Read the model definition and answer for the solid it produces. Units are mm, in the model's axes. Coordinates: 2 decimals unless noted, no trailing zeros. Order: outer loops, then holes, each group sorted by start corner. A loop starts at its lowest first (then second) coordinate and runs counter-clockwise, first axis right, second up. Notation, with made-up numbers: (64.25, 87) -> (112.25, 87) arc R31 ccw to (112.25, 115) -> close; hole circle Ø1 at (70.25, -30.75). An arc over 180 degrees is marked (long way). Answer in a Markdown table with one row per item.
from build123d import *

# Parameters (mm, degrees)
REVOLVE3_ANGLE      = 90
BOSS_EXTRUDE2_DEPTH = 1000


with BuildPart() as part:
    # Sketch2 → Revolve3 (revolve)
    with BuildSketch(Plane.XY):
        with BuildLine():
            Line((-0.654182434, 15.02), (-10.654182434, 15.02))
            Line((-10.654182434, 15.02), (-10.654182434, 0))
            Line((-10.654182434, 0), (0, 0))
            Line((0, 0), (25.4, 0))
            Line((25.4, 0), (35.4, 0))
            Line((35.4, 0), (35.4, 4.5))
            Line((35.4, 4.5), (25.4, 4.5))
            add(Edge.make_bspline(
                [(-0.654182434, 15.02), (-0.219836229, 14.810704372), (0.610598489, 14.410982375), (2.74095302, 13.386545583), (4.34709547, 12.619135975), (6.701613478, 11.49599419), (8.606916476, 10.59589253), (10.790885987, 9.570629713), (12.810835282, 8.63757915), (14.944119423, 7.669787097), (16.950761864, 6.79193378), (18.75556814, 6.044207346), (20.238794329, 5.486207444), (21.39416777, 5.103578745), (22.215591012, 4.870934478), (22.897035956, 4.710298297), (23.464492683, 4.605633048), (23.954091395, 4.538072471), (24.354277235, 4.503624983), (24.669284768, 4.488813447), (24.918595629, 4.485402054), (25.124701431, 4.488218611), (25.279381224, 4.493757229), (25.359889237, 4.497669109), (25.4, 4.5)],
                knots=[0.083771138, 0.083771138, 0.083771138, 0.083771138, 0.083771138, 0.152014176, 0.220257214, 0.288500251, 0.356743288, 0.424986327, 0.493229366, 0.561472406, 0.629715448, 0.697958493, 0.757156968, 0.791278497, 0.81934393, 0.841893906, 0.858954658, 0.874282948, 0.887931591, 0.900718778, 0.906405686, 0.912092593, 0.917779499, 0.923466404, 0.923466404, 0.923466404, 0.923466404, 0.923466404], degree=4))
        make_face()
    revolve(axis=Axis((0, 0, 0), (1, 0, 0)), revolution_arc=REVOLVE3_ANGLE)

    # Sketch11 → Boss-Extrude2 (add)
    with BuildSketch(Plane.XY):
        with BuildLine():
            Line((25.133318649, 0), (101.333318649, 0))
            ThreePointArc((101.333318649, 0), (63.233318649, 38.1), (25.133318649, 0))
        make_face()
    extrude(amount=BOSS_EXTRUDE2_DEPTH)


solid = part.part
Q1. Given pin 1 (5 mm diameter, centred on y = 6, z = 335.5, fed in from +X); pin 2 (12 mm diameter, centred on x = 67.5, z = 570.5, fed in from +Y); pin 3 (8 mm diameter, centred on x = 52, z = 739.5, fed in from +Y), each flat-ended and moving along its own axis, determine where each tip first touches the part or whether it passes through.
Outcome:
| item | result |
|---|---|
| pin 1 | x = 101.17 |
| pin 2 | y = 38.1 |
| pin 3 | y = 37.41 |
Q2. The part is cut by section A-A (z = 454). Write down the section's boundary in (x, y).
Outcome:
| item | result |
|---|---|
| outline | (25.13, 0) -> (101.33, 0) arc R38.1 ccw to start |
Q3. The part is cut by section C-C (y = 31.5). Write down the section's boundary in (x, z), then the cut area to 3 significant figures.
Outcome:
| item | result |
|---|---|
| outline | (41.8, 0) -> (84.67, 0) -> (84.67, 1000) -> (41.8, 1000) -> close |
| area | 42,900 mm² |
Q4. For a pull along Z with two mould halves and no side action, classify faces 1 (the face through (63, 15, 1000)), 2 (the face through (57, 15, 0)), 3 (the face through (64.07, 38.09, 493)) as pulls with the +Z half, pulls with the -Z half, needs draft (parallel to the pull), parting line crosses it, or undercut.
Outcome:
| item | result |
|---|---|
| face 1 | pulls with the +Z half |
| face 2 | pulls with the -Z half |
| face 3 | needs draft |
Q5. Consider line 1 (Y direction, x = 61, z = 574); line 2 (Y direction, x = 61.5, z = 327); line 3 (X direction, y = 7.5, z = 498.5). Determine where each line is inside the solid, lowest interval first.
Outcome:
| item | result |
|---|---|
| line 1 | 0 to 38.03 |
| line 2 | 0 to 38.06 |
| line 3 | 25.88 to 100.59 |
Q6. The part is cut by section B-B (x = 70.5). Write down the section's boundary in (y, z), then the cut area to 3 significant figures.
Outcome:
| item | result |
|---|---|
| outline | (0, 0) -> (37.4, 0) -> (37.4, 1000) -> (0, 1000) -> close |
| area | 37,400 mm² |
